Read the model definition and answer for the solid it produces. Units are mm, in the model's axes. A direction names the side the tool comes from. Round coordinates to 2 decimals unless told otherwise and drop trailing zeros. Answer as CSV lines item,"result". Start each with the question number.
1) Which of the six approach directions +Z, -Z, +X, -X, +Y, -Y give full straight-line access (tool end or side, diameter ignored) to faces 1 (the flat face through (54, 10, -15)), 2 (the flat face through (30, 0, -20))?
2) For a pull along Z with two mould halves and no side action, classify faces 3 (the flat face through (60, 6, -29)), 4 (the flat face through (35, 25, -15)), 5 (the flat face through (30, 20, -40)) as +Z half, -Z half, draft (parallel to the pull), parting line (faces both ways), or undercut.
3) Each of these flat-tipped pins is pushed along its axis until it touches: pin 1 (15 mm diameter, centred on x = 43.5, z = -13.5, fed in from +Y); pin 2 (5 mm diameter, centred on x = 48, z = -14.5, fed in from +Y). Where does it stop, or does it pass through?
4) Consider line 1 along Y through (x, z) = (56.5, -28); line 2 along Z through (x, y) = (51.5, 36); line 3 along X through (y, z) = (35.5, -8.5). Determine where each line is inside the solid, lowest interval first.
Autodesk Inventor part; units mm, degrees
ref_plane "工作平面1" through (20, 40, 0) normal (-0.8018, -0.5345, -0.2673) x (0.3162, 0, -0.9487)
ref_plane "YZ Plane" through (0, 0, 0) normal (1, 0, 0) x (0, 1, 0)
ref_plane "XZ Plane" through (0, 0, 0) normal (0, 1, 0) x (-1, 0, 0)
sketch "草圖1" plane through (0, 0, 0) normal (0, 1, 0) x (-1, 0, 0)
  line L0 (0, 0) -> (-60, 0)
  line L1 (-60, 0) -> (-60, -40)
  line L2 (-60, -40) -> (0, -40)
  line L3 (0, -40) -> (0, 0)
  dimension "d0" = 40
  dimension "d1" = 60
extrude "擠出1" add sketch "草圖1" along normal blind 10
sketch "草圖2" plane through (0, 10, 0) normal (0, 1, 0) x (1, 0, 0)
  line L0 (0, 0) -> (60, 0)
  line L1 (20, 0) -> (30, 30)
  line L2 (30, 30) -> (60, 30)
  line L3 (60, 0) -> (60, 40)
  line L4 (60, 30) -> (60, 40)
  line L5 (60, 40) -> (0, 40)
  line L6 (60, 40) -> (0, 40)
  line L7 (0, 40) -> (0, 0)
  line L8 (20, 0) -> (0, 0)
  dimension "d4" = 10
  dimension "d5" = 30
  dimension "d6" = 30
extrude "擠出2" add sketch "草圖2" along normal blind 30 contours L7 L5 L3 L2 L1 L0
sketch "草圖3" plane through (0, 10, 0) normal (0, 1, 0) x (1, 0, 0)
  line L0 (0, 0) -> (60, 0)
  line L1 (40, 0) -> (50, 30)
  line L2 (30, 30) -> (60, 30)
  dimension "d9" = 10
  dimension "d10" = 20
ref_plane "工作平面1" through (20, 40, 0) normal (-0.8018, -0.5345, -0.2673) x (0.3162, 0, -0.9487)
sketch "草圖4" plane through (20, 40, 0) normal (-0.8018, -0.5345, -0.2673) x (0.3162, 0, -0.9487)
  line L0 (31.6228, 25.3546) -> (0, 25.3546)
  line L1 (31.6228, 25.3546) -> (31.6228, 0)
  line L2 (0, 0) -> (31.6228, 0)
  line L3 (0, 25.3546) -> (0, 0)
  line L4 (41.1096, 40.5674) -> (31.6228, 25.3546)
  line L5 (31.6228, 25.3546) -> (0, 25.3546)
  line L6 (0, 25.3546) -> (12.6491, 45.6383)
  line L7 (12.6491, 45.6383) -> (41.1096, 40.5674)
  line L8 (6.3246, 35.4965) -> (37.9473, 35.4965)
  line L9 (37.9473, 35.4965) -> (31.6228, 0)
  line L10 (31.6228, 0) -> (41.1096, 15.2128)
  line L11 (31.6228, 0) -> (31.6228, 25.3546)
  line L12 (37.9473, 35.4965) -> (31.6228, 25.3546)
  point P0 (-6.3246, 23.6643)
extrude "擠出3" add sketch "草圖4" along normal up to next contours L1 L2 L3 L0 | L4 L9 L1 | L0 L6 L8 L4
sketch "草圖5" plane through (0, 0, 0) normal (0, 0, 1) x (1, 0, 0)
  line L0 (-0.672, 48.4854) -> (66.1118, 48.4854)
  line L1 (66.1118, 48.4854) -> (66.1118, -3.1014)
  line L2 (66.1118, -3.1014) -> (-0.672, -3.1014)
  line L3 (-0.672, -3.1014) -> (-0.672, 48.4854)
  point P0 (0, 0)
extrude "擠出4" cut sketch "草圖5" along normal blind 30
properties part number "49"
Check values:
1,face 1,"+Z, +X, +Y"
1,face 2,"+Z, -Z, +X, -X, -Y"
2,face 3,"draft"
2,face 4,"+Z half"
2,face 5,"-Z half"
3,pin 1,"stops at y = 23.36"
3,pin 2,"stops at y = 10"
4,line 1,"y = 0 to 10"
4,line 2,"z = -40 to -30"
4,line 3,"x = 0 to 25.83"
